Check sheet for the modelled part. Datum: model origin and axes. Units: mm. A direction names the side the tool comes from. Round coordinates to 2 decimals unless told otherwise and drop trailing zeros. Write each loop counter-clockwise with the first axis right and the second up, starting at its lowest first coordinate (ties: lowest second). Pieces come first, ordered by that corner, then holes. Notation, with made-up numbers: (68.25, 6.25) -> (83.25, 6.25) arc R28 ccw to (83.25, 45.25) -> close; hole circle Ø3 at (6, 70.5). An arc over 180 degrees is marked (long way). Write item = value, one per line.
from build123d import *

# Parameters (mm, degrees)
ESQUISSE1_W             = 10
ESQUISSE1_H             = 600
BOSS_EXTRU_1_DEPTH      = 129.973967
ENL_V_MAT_EXTRU_1_DEPTH = 10


with BuildPart() as part:
    # Esquisse1 → Boss.-Extru.1 (new body)
    with BuildSketch(Plane.XY):
        with Locations((-160.641983179, 300)):
            Rectangle(ESQUISSE1_W, ESQUISSE1_H)
    extrude(amount=BOSS_EXTRU_1_DEPTH)

    # Esquisse2 → Enlèv. mat.-Extru.1 (cut)
    with BuildSketch(Plane(origin=(-155.641983179, 0, 0), x_dir=(0, 0, -1), z_dir=(1, 0, 0))):
        with BuildLine():
            Line((0, 600), (-75.04598428, 600))
            Line((-75.04598428, 600), (-75.04598428, 450))
            ThreePointArc((-75.04598428, 450), (-72.117052092, 442.928932188), (-65.04598428, 440))
            Line((-65.04598428, 440), (0, 440))
            Line((0, 440), (0, 600))
        make_face()
    extrude(amount=-ENL_V_MAT_EXTRU_1_DEPTH, mode=Mode.SUBTRACT)


solid = part.part
(1) Material ranges on L1, parallel to Y at x = -157.25, z = 7.5; L2, parallel to Z at x = -161, y = 484.5, recorded low to high. Write a range as [from, to].
Worked answers:
L1 = [0, 440]
L2 = [75.05, 129.97]
(2) Sectioned sample at A-A on x = -159. Enter the section's corners in (y, z).
Worked answers:
outline = (0, 0) -> (440, 0) -> (440, 65.05) arc R10 cw to (450, 75.05) -> (600, 75.05) -> (600, 129.97) -> (0, 129.97) -> close
(3) Release check for a two-part mould opening along Y. For faces 1 (the flat face through (-161, 0, 64)), 2 (the flat face through (-161, 304, 129.974)), 3 (the flat face through (-161, 440, 33)) record: pulls with the +Y half, pulls with the -Y half, needs draft (parallel to the pull), parting line crosses it, or undercut.
Worked answers:
face_1 = pulls with the -Y half
face_2 = needs draft
face_3 = pulls with the +Y half
(4) Go/stop test with flat-tipped pins: P1, Ø4, axis at x = -157, z = 22.5, coming from the +Y side; P2, Ø6, axis at x = -158.5, z = 25, coming from the -Y side. Record where each tip stops, or that it passes through.
Worked answers:
P1 = 440
P2 = 0
(5) Access from +Z, -Z, +X, -X, +Y, -Y to the whole of each face (thin tool, end or side, straight path). Record for faces 4 (the flat face through (-161, 223, 0)), 5 (the flat face through (-161, 526, 75.046)).
Worked answers:
face_4 = -Z, +X, -X, +Y, -Y
face_5 = -Z, +X, -X, +Y
(6) Sectioned sample at B-B on z = 45. Enter the section's corners in (x, y), then the cut area to 3 significant figures.
Worked answers:
outline = (-165.64, 0) -> (-155.64, 0) -> (-155.64, 440) -> (-165.64, 440) -> close
area = 4,400 mm²
